Autodesk Inventor part; units mm, degrees
ref_plane "YZ Plane" through (0, 0, 0) normal (1, 0, 0) x (0, 1, 0)
ref_plane "XZ Plane" through (0, 0, 0) normal (0, 1, 0) x (-1, 0, 0)
ref_plane "XY Plane" through (0, 0, 0) normal (0, 0, 1) x (1, 0, 0)
sketch "スケッチ1" plane through (0, 0, 0) normal (0, 1, 0) x (-1, 0, 0)
  line L0 (180, 60) -> (-180, 60)
  line L1 (-180, 60) -> (-180, -60)
  line L2 (-180, -60) -> (180, -60)
  line L3 (180, -60) -> (180, 60)
  line L4 (180, 60) -> (-180, -60) construction
  line L5 (-180, 60) -> (180, -60) construction
  line L6 (180, 57) -> (-180, 57)
  line L7 (-60, 60) -> (-60, -60)
  line L8 (-60, 40) -> (-80, 40)
  line L9 (-80, 40) -> (-80, 20)
  line L10 (-80, 20) -> (-60, 20)
  line L11 (252, 0) -> (-252, 0) construction
  line L12 (-60, -40) -> (-80, -40)
  line L13 (-80, -40) -> (-80, -20)
  line L14 (-80, -20) -> (-60, -20)
  line L15 (0, -84) -> (0, 84) construction
  line L16 (60, 60) -> (60, -60)
  line L17 (60, 40) -> (80, 40)
  line L18 (80, 40) -> (80, 20)
  line L19 (80, 20) -> (60, 20)
  line L20 (60, -40) -> (80, -40)
  line L21 (80, -20) -> (60, -20)
  line L22 (80, -40) -> (80, -20)
  line L23 (-60, 19.7) -> (-80.3, 19.7)
  line L24 (-80.3, 19.7) -> (-80.3, 40.3)
  line L25 (-80.3, 40.3) -> (-60, 40.3)
  line L26 (-60, -19.7) -> (-80.3, -19.7)
  line L27 (-80.3, -19.7) -> (-80.3, -40.3)
  line L28 (-80.3, -40.3) -> (-60, -40.3)
  line L29 (60, 19.7) -> (80.3, 19.7)
  line L30 (80.3, 19.7) -> (80.3, 40.3)
  line L31 (80.3, 40.3) -> (60, 40.3)
  line L32 (60, -19.7) -> (80.3, -19.7)
  line L33 (80.3, -19.7) -> (80.3, -40.3)
  line L34 (80.3, -40.3) -> (60, -40.3)
  point P0 (0, 0)
  point P1 (-60, 57)
  dimension "d0" = 120
  dimension "d1" = 360
  dimension "d4" = 3
  dimension "d5" = 120
  dimension "d7" = 20
  dimension "d8" = 20
  dimension "d9" = 20
  dimension "d10" = 0.3
  dimension "d11" = 0.3
extrude "押し出し3" add sketch "スケッチ1" along normal blind 25 contours L3 L6 L16 L0 | L16 L6 L7 L0 | L7 L6 L1 L0
extrude "押し出し1" add sketch "スケッチ1" along normal blind 2 contours L7 L6 L1 L0 | L7 L25 L24 L23 L26 L27 L28 L2 L1 L6 | L7 L8 L9 L10 L23 L24 L25 | L7 L10 L9 L8 | L28 L27 L26 L7 L14 L13 L12 | L12 L13 L14 L7
extrude "押し出し2" cut sketch "スケッチ1" against normal blind 1 from surface at 2 contours L7 L10 L9 L8 | L12 L13 L14 L7
sketch "スケッチ2" plane through (-180, 0, 60) normal (0, 0, 1) x (1, 0, 0)
  line L0 (0, 0) -> (360, 0)
  line L1 (360, 0) -> (360, 25)
  line L2 (0, 25) -> (360, 25)
  line L3 (0, 0) -> (0, 25)
  line L4 (240, 0) -> (240, 25)
  line L5 (240, 7.5) -> (255, 7.5)
  line L6 (255, 7.5) -> (255, 17.5)
  line L7 (255, 17.5) -> (240, 17.5)
  line L8 (180, -5) -> (180, 30) construction
  line L9 (120, 0) -> (120, 25)
  line L10 (120, 7.5) -> (105, 7.5)
  line L11 (105, 7.5) -> (105, 17.5)
  line L12 (105, 17.5) -> (120, 17.5)
  line L13 (240, 17.9) -> (255.4, 17.9)
  line L14 (255.4, 17.9) -> (255.4, 7.1)
  line L15 (255.4, 7.1) -> (240, 7.1)
  line L16 (120, 17.9) -> (104.6, 17.9)
  line L17 (104.6, 17.9) -> (104.6, 7.1)
  line L18 (104.6, 7.1) -> (120, 7.1)
  point P0 (180, 0)
  point P1 (360, 12.5)
  dimension "d16" = 120
  dimension "d17" = 10
  dimension "d18" = 15
  dimension "d19" = 7.5
  dimension "d24" = 0.4
extrude "押し出し4" cut sketch "スケッチ2" against normal blind 25 contours L3 L2 L9 L16 L17 L18 L0 | L9 L2 L4 L0 | L18 L17 L16 L9 L12 L11 L10 | L10 L11 L12 L9
extrude "押し出し5" cut sketch "スケッチ2" against normal blind 1.5 contours L4 L5 L6 L7 L13 L14 L15 | L4 L7 L6 L5
fillet "フィレット2" radius 4 1 edges at (120, 2, 57)
fillet "フィレット3" radius 1 3 edges at (180, 15.5, 57) (180, 2, -3.5) (120, 2, -60)
properties part number "protectar1"
Can you work these out from the model? Positions are in its coordinate system, mm. A direction names the side the tool comes from. Coordinates: 2 decimals unless noted, no trailing zeros. Write each loop counter-clockwise with the first axis right and the second up, starting at its lowest first coordinate (ties: lowest second). Pieces come first, ordered by that corner, then holes. Notation, with made-up numbers: (50, -16) -> (73, -16) arc R13 cw to (73, 5) -> close; hole circle Ø11 at (25, -31). An arc over 180 degrees is marked (long way). Answer as CSV lines item,"result".
1) On a 3-axis mill with a long thin cutter (end or side, diameter ignored), from which of +Z, -Z, +X, -X, +Y, -Y can I reach the whole of each face in a straight line? I mean faces 1 (the flat face through (68, 13, 58.5)), 2 (the flat face through (180, 0.4, 26.9)), 3 (the flat face through (119, 15, 57)), 4 (the flat face through (70, 1, -30)), 5 (the flat face through (60, 0.4, 22.5)). Say none if no direction works.
Check result:
face 1,"+Z, -X"
face 2,"+Z, -Z, +X, +Y, -Y"
face 3,"-Z, +X, -X, +Y"
face 4,"-X, +Y"
face 5,"+Z, -Z, -X, +Y, -Y"
2) If we section it at A-A on z = -33: Please give me the cut outline in (x, y), then the cut area to 3 significant figures.
Check result:
outline,"(60, 0) -> (180, 0) -> (180, 1) arc R1 ccw to (179, 2) -> (80, 2) -> (80, 1) -> (60, 1) -> close"
area,"220 mm²"
3) If I drill on line 1 (Z direction, x = 113, y = 19.75); line 2 (Y direction, x = 94.5, z = -28.5); line 3 (Z direction, x = 68.5, y = 13.5), over which ranges is the centre line in solid material (lowest first)? Write a range as from..to.
Check result:
line 1,"57..60"
line 2,"0..2"
line 3,"57..58.5"
4) If we section it at B-B on x = 143: Please give me the cut outline in (y, z), then the cut area to 3 significant figures.
Check result:
outline,"(0, -60) -> (1, -60) arc R1 ccw to (2, -59) -> (2, 53) arc R4 cw to (6, 57) -> (25, 57) -> (25, 60) -> (0, 60) -> close"
area,"312 mm²"
5) If we mould it in two halves opening along Z, with no side actions, what happens to faces 6 (the flat face through (119, 12, 60)), 7 (the flat face through (70, 1, 30)), 8 (the flat face through (120, 2, -2))? For each: +Z half, -Z half, draft (parallel to the pull), parting line (faces both ways), or undercut.
Check result:
face 6,"+Z half"
face 7,"undercut"
face 8,"draft"
6) If we section it at D-D on y = 20.5: Please give me the cut outline in (x, z), then the cut area to 3 significant figures.
Check result:
outline,"(60, 57) -> (179, 57) arc R1 ccw to (180, 58) -> (180, 60) -> (60, 60) -> close"
area,"360 mm²"
7) If we section it at C-C on y = 10.5: Please give me the cut outline in (x, z).
Check result:
outline,"(60, 57) -> (179, 57) arc R1 ccw to (180, 58) -> (180, 60) -> (75.4, 60) -> (75.4, 58.5) -> (60, 58.5) -> close"
8) Will these pins go through, and if not, where does the flat tip stop? P1, Ø5.5, axis at x = 143.5, y = 14, coming from the -Z side; P2, Ø0.8, axis at x = 73.5, y = 1.5, coming from the -Z side (3 decimals); P3, Ø6, axis at x = 132.5, z = 18.5, coming from the -Y side; P4, Ø10, axis at x = 73, z = 29, coming from the +Y side.
Check result:
P1,"z = 57"
P2,"z = -59.995"
P3,"y = 0"
P4,"y = 1"
